```python
from build123d import *

# Parameters (mm, degrees)
F0_W     = 750
F0_H     = 2300
F1_DEPTH = 18
F2_R     = 15
F4_D     = 8
F4_DEPTH = 15
F4_TIP   = 2.4034424761
F5_R     = 40
F6_DEPTH = 18


with BuildPart() as f1:
    # F0 (on Top) → F1 (new body)
    with BuildSketch(Plane.XY):
        with Locations((375, -1150)):
            Rectangle(F0_W, F0_H)
    extrude(amount=F1_DEPTH)

    # F2
    f2_edges = [f1.edges().sort_by_distance(p)[0] for p in [
        (0, -2300, 9),
        (750, -2300, 9),
    ]]
    fillet(f2_edges, radius=F2_R)

    # F4
    with Locations(Plane(origin=(0, 0, 0), x_dir=(1, 0, 0), z_dir=(0, 0, -1))):
        with Locations((500, 100), (250, 100), (500, 2200), (500, 2100), (250, 2200), (250, 2100), (250, 1850), (500, 1850), (250, 1600), (500, 1600), (500, 1350), (250, 1350), (500, 1100), (250, 1100), (500, 850), (250, 850), (250, 600), (500, 600), (500, 350), (250, 350), (375, 100), (375, 350), (375, 600), (375, 850), (375, 1100), (375, 1350), (375, 1600), (375, 1850), (375, 2100), (643.933982822, 106.066017178), (467.1572875254, 282.8427124746), (639.5405845398, 2189.5405845398), (462.7638892432, 2012.7638892432)):
            Hole(F4_D / 2, depth=F4_DEPTH)
            with Locations((0, 0, -(F4_DEPTH + F4_TIP / 2))):  # 118° drill point
                Cone(0, F4_D / 2, F4_TIP, mode=Mode.SUBTRACT)

    # F5 (on face) → F6 (cut)
    with BuildSketch(Plane(origin=(0, 0, 0), x_dir=(1, 0, 0), z_dir=(0, 0, -1))):
        with Locations((630, 300)):
            Circle(F5_R)
        with Locations((620, 2000)):
            Circle(F5_R)
        with Locations((630, 1150)):
            Circle(F5_R)
    extrude(amount=-F6_DEPTH, mode=Mode.SUBTRACT)


solid = f1.part
```
The listing builds one solid part. Answer for the finished solid, in the listing's coordinates (mm). Give positions to 0.01 mm unless a question says otherwise; leave off trailing zeros. Answer as a JSON object with one key per item and string values. Group by question number.
Item 1: Flat-ended cylindrical pins translate along their axes: pin 1 (5 mm diameter, centred on x = 500, y = -850, fed in from -Z); pin 2 (6.5 mm diameter, centred on x = 250, y = -350, fed in from -Z); pin 3 (7 mm diameter, centred on x = 375, y = -350, fed in from -Z). Find the tip coordinate at first contact, or state that the pin passes through.
Item 2: Consider L1, parallel to X at y = -850, z = 4.25; L2, parallel to X at y = -1602, z = 6; L3, parallel to Y at x = 665, z = 12.5. Determine where each line is inside the solid, lowest interval first. Write a range as from..to.
Item 3: Determine the mould class of faces 1 (the flat face through (370, -1134, 0)), 2 (the cylindrical face through (614.79, -2039.66, 8.87)) for opening direction X: pulls with the +X half, pulls with the -X half, needs draft (parallel to the pull), parting line crosses it, or undercut.
Result set:
{
 "1": {"pin 1": "z = 15.9", "pin 2": "z = 15.45", "pin 3": "z = 15.3"},
 "2": {"L1": "0..246, 254..371, 379..496, 504..750", "L2": "0..246.54, 253.46..371.54, 378.46..496.54, 503.46..750", "L3": "-2300..-1169.36, -1130.64..-319.36, -280.64..0"},
 "3": {"face 1": "needs draft", "face 2": "undercut"}
}
